Here's how the part is built. I have some questions about the finished solid (model axes, mm). Round coordinates to 2 decimals unless told otherwise and drop trailing zeros. Loops run counter-clockwise (first coordinate to the right, second up) from the corner with the lowest first, then second, coordinate; pieces in that order, holes last. Notation, with made-up numbers: (0.25, 33) - (42.25, 33) arc R24 ccw to (42.25, 49) - close; hole circle Ø7 at (73, 16.5). An arc over 180 degrees is marked (long way). Answer as a JSON object with one key per item and string values. Group by question number.
1) I want a section at C-C, the plane z = -3. Please give me the cut outline in (x, y), then the cut area to 3 significant figures.
2) I want a section at B-B, the plane x = 28.5. Please give me the cut outline in (y, z).
3) If I drill on line 1 along Y through (x, z) = (-25, -2.75); line 2 along X through (y, z) = (-28.5, -3.5); line 3 along X through (y, z) = (-24.5, -8), over which ranges is the centre line in solid material (lowest first)? Write a range as [from, to].
4) I want a section at D-D, the plane y = -31.75. Please give me the cut outline in (x, z), then the cut area to 3 significant figures.
5) If we mould it in two halves opening along X, with no side actions, what happens to faces 1 (the face through (24.46, -24.185, -5.226)), 2 (the face through (-25.54, -24.185, -5.226)), 3 (the face through (0, -28, -10.6))? For each: pulls with the +X half, pulls with the -X half, needs draft (parallel to the pull), parting line crosses it, or undercut.
6) I want a section at A-A, the plane y = -28.3. Please give me the cut outline in (x, z).
7) Will these pins go through, and if not, where does the flat tip stop? P1, Ø1, axis at y = -25.5, z = -6, coming from the -X side; P2, Ø5, axis at y = -27.5, z = -7, coming from the +X side.
from build123d import *

# Parameters (mm, degrees)
SKETCH1_R           = 4.15
BOSS_EXTRUDE2_DEPTH = 10.6


with BuildPart() as part:
    # Sketch1 → Boss-Extrude2 (new body)
    with BuildSketch(Plane.XY):
        with BuildLine():
            Line((-25, -36.3), (25, -36.3))
            ThreePointArc((25, -36.3), (32.292866569, -31.588479467), (30.995610492, -23.003524301))
            ThreePointArc((30.995610492, -23.003524301), (28.288479467, -21.007133431), (25, -20.3))
            Line((25, -20.3), (-25, -20.3))
            ThreePointArc((-25, -20.3), (-28.288479467, -21.007133431), (-30.995610492, -23.003524301))
            ThreePointArc((-30.995610492, -23.003524301), (-32.292866569, -31.588479467), (-25, -36.3))
        make_face()
        with Locations((-25, -28.3)):
            Circle(SKETCH1_R, mode=Mode.SUBTRACT)
        with Locations((25, -28.3)):
            Circle(SKETCH1_R, mode=Mode.SUBTRACT)
    extrude(amount=-BOSS_EXTRUDE2_DEPTH)


solid = part.part
Outcome:
{
 "1": {"outline": "(-25, -36.3) - (25, -36.3) arc R8 ccw to (25, -20.3) - (-25, -20.3) arc R8 ccw to start; hole circle Ø8.3 at (-25, -28.3); hole circle Ø8.3 at (25, -28.3)", "area": "893 mm^2"},
 "2": {"outline": "(-35.49, -10.6) - (-30.53, -10.6) - (-30.53, 0) - (-35.49, 0) - close; (-26.07, -10.6) - (-21.11, -10.6) - (-21.11, 0) - (-26.07, 0) - close"},
 "3": {"line 1": "[-36.3, -32.45], [-24.15, -20.3]", "line 2": "[-33, -29.15], [-20.85, 20.85], [29.15, 33]", "line 3": "[-32.04, -26.67], [-23.33, 23.33], [26.67, 32.04]"},
 "4": {"outline": "(-32.22, -10.6) - (-27.31, -10.6) - (-27.31, 0) - (-32.22, 0) - close; (-22.69, -10.6) - (22.69, -10.6) - (22.69, 0) - (-22.69, 0) - close; (27.31, -10.6) - (32.22, -10.6) - (32.22, 0) - (27.31, 0) - close", "area": "585 mm^2"},
 "5": {"face 1": "undercut", "face 2": "undercut", "face 3": "needs draft"},
 "6": {"outline": "(-33, -10.6) - (-29.15, -10.6) - (-29.15, 0) - (-33, 0) - close; (-20.85, -10.6) - (20.85, -10.6) - (20.85, 0) - (-20.85, 0) - close; (29.15, -10.6) - (33, -10.6) - (33, 0) - (29.15, 0) - close"},
 "7": {"P1": "x = -32.66", "P2": "x = 33"}
}
